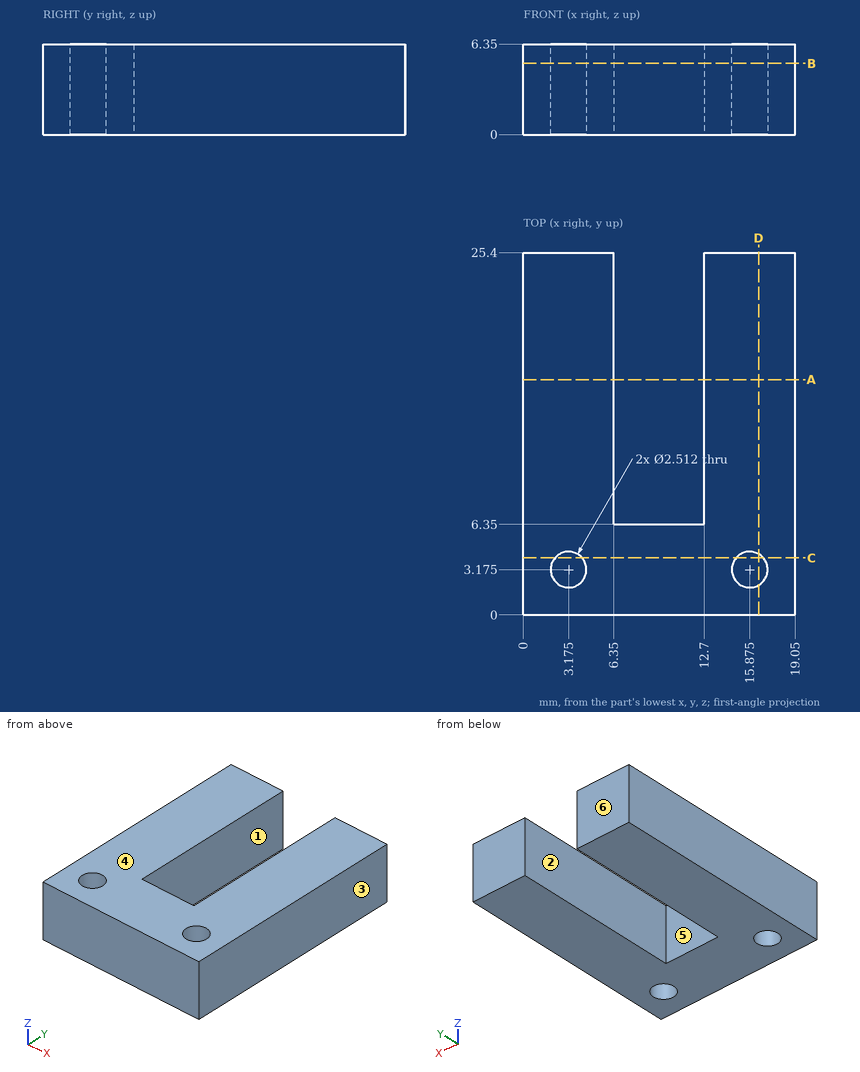
Check sheet for the drawn part. Datum: minimum x, y, z corner. Units: mm. A direction names the side the tool comes from. Round coordinates to 2 decimals unless told otherwise and drop trailing zeros. Loops run counter-clockwise (first coordinate to the right, second up) from the corner with the lowest first, then second, coordinate; pieces in that order, holes last. Notation, with made-up numbers: (-22, 22.25) - (18, 22.25) arc R19 cw to (18, 42.25) - close; hole circle Ø5 at (36.5, 22). An arc over 180 degrees is marked (long way). Answer as a JSON object with one key per item and string values. Group by question number.
Q1. Scan lines: line 1 along X through (y, z) = (22, 6); line 2 along Y through (x, z) = (3.25, 4.75); line 3 along X through (y, z) = (3.75, 5.25). Record each from-to range of solid material in increasing order. Write a range as [from, to].
Q2. Mould release check, pull along X, two halves, no side actions. Record for the marked faces 1, 2, 3 and 4: released by +X, released by -X, zero draft, split by the parting line, or undercut.
Q3. Set-up check for the marked faces 5 and 6: record each of +Z, -Z, +X, -X, +Y, -Y from which the full face is reachable in a straight line by a thin tool's end or side.
Q4. Sectioned sample at A-A, the plane y = 16.5. Enter the section's corners in (x, z).
Q5. Sectioned sample at C-C, the plane y = 4. Enter the section's corners in (x, z).
Q6. Sectioned sample at D-D, the plane x = 16.5. Enter the section's corners in (y, z).
Q7. Sectioned sample at B-B, the plane z = 5. Enter the section's corners in (x, y) (3 decimals).
Solution:
{
 "1": {"line 1": "x = [0, 6.35], [12.7, 19.05]", "line 2": "y = [0, 1.92], [4.43, 25.4]", "line 3": "x = [0, 2.06], [4.29, 14.76], [16.99, 19.05]"},
 "2": {"face 1": "undercut", "face 2": "undercut", "face 3": "released by +X", "face 4": "zero draft"},
 "3": {"face 5": "+Z, -Z, +Y", "face 6": "+Z, -Z, +X, -X, +Y"},
 "4": {"outline": "(0, 0) - (6.35, 0) - (6.35, 6.35) - (0, 6.35) - close; (12.7, 0) - (19.05, 0) - (19.05, 6.35) - (12.7, 6.35) - close"},
 "5": {"outline": "(0, 0) - (2.23, 0) - (2.23, 6.35) - (0, 6.35) - close; (4.12, 0) - (14.93, 0) - (14.93, 6.35) - (4.12, 6.35) - close; (16.82, 0) - (19.05, 0) - (19.05, 6.35) - (16.82, 6.35) - close"},
 "6": {"outline": "(0, 0) - (2.09, 0) - (2.09, 6.35) - (0, 6.35) - close; (4.26, 0) - (25.4, 0) - (25.4, 6.35) - (4.26, 6.35) - close"},
 "7": {"outline": "(0, 0) - (19.05, 0) - (19.05, 25.4) - (12.7, 25.4) - (12.7, 6.35) - (6.35, 6.35) - (6.35, 25.4) - (0, 25.4) - close; hole circle Ø2.512 at (3.175, 3.175); hole circle Ø2.512 at (15.875, 3.175)"}
}
